from build123d import *

# Parameters (mm, degrees)
EXTRUDE_1_DEPTH = 7.65
SKETCH_2_R      = 6
EXTRUDE_2_DEPTH = 30
FILLET_1_R      = 0.6


with BuildPart() as part:
    # 草图1 → 凸台-拉伸1 (new body)
    with BuildSketch(Plane(origin=(0, 0, 0), x_dir=(1, 0, 0), z_dir=(0, 1, 0))):
        Polygon((6.921438907, -7.752011575), (10.174158408, 2.118136136), (3.252719501, 9.870147711), (-6.921438907, 7.752011575), (-10.174158408, -2.118136136), (-3.252719501, -9.870147711), align=None)
    extrude(amount=EXTRUDE_1_DEPTH)

    # 草图2 → 凸台-拉伸2 (add)
    with BuildSketch(Plane.XZ):
        Circle(SKETCH_2_R)
    extrude(amount=EXTRUDE_2_DEPTH)

    # 圆角1
    fillet_1_edges = [part.edges().sort_by_distance(p)[0] for p in [
        (6.713438955, 7.65, -5.994141924),
        (-1.834359703, 7.65, -8.811079643),
        (-8.547798657, 7.65, -2.81693772),
        (-6.713438955, 7.65, 5.994141924),
        (1.834359703, 7.65, 8.811079643),
        (8.547798657, 7.65, 2.81693772),
    ]]
    fillet(fillet_1_edges, radius=FILLET_1_R)


solid = part.part
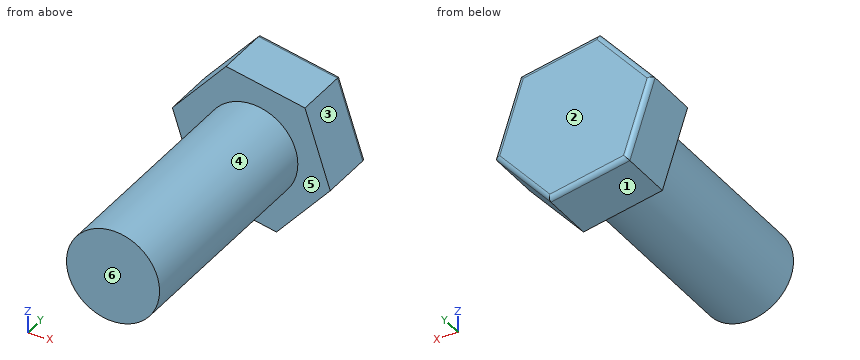
Can you work these out from the model? Positions are in its coordinate system, mm. Face numbers are marked on the shaded views. A direction names the side the tool comes from. Round coordinates to 2 decimals unless told otherwise and drop trailing zeros. Order: outer loops, then holes, each group sorted by start corner. A loop starts at its lowest first (then second) coordinate and runs counter-clockwise, first axis right, second up. Notation, with made-up numbers: (72.5, 40.5) -> (124.5, 40.5) arc R20 ccw to (124.5, 47.5) -> close; hole circle Ø10 at (16, 37.5). An arc over 180 degrees is marked (long way). Write each question's results on one line, items separated by ' | '. Start each with the question number.
Item 1: Will these pins go through, and if not, where does the flat tip stop? pin 1 (1 mm diameter, centred on y = -24, z = 2, fed in from +X); pin 2 (8 mm diameter, centred on y = -17, z = -5, fed in from +X); pin 3 (2 mm diameter, centred on x = -5, y = -4, fed in from -Z).
Item 2: Thinking about a two-plate mould opening in Z: for the marked faces 1, 2, 3 and 4, which applies, +Z half, -Z half, draft (parallel to the pull), parting line (faces both ways), or undercut?
Item 3: Which directions (+Z, -Z, +X, -X, +Y, -Y) give clear straight access to the entire face, cutting with the end or side of a thin tool? Please do the marked faces 5 and 6.
Item 4: If we section it at A-A, the plane y = 2: Write out the boundary of the cut face in (x, z), then the cut area to 3 significant figures.
Item 5: Please list where these lines run through material, in increasing order: L1, parallel to Y at x = 8, z = 2.75; L2, parallel to X at y = -26, z = 1.25; L3, parallel to Z at x = 6, y = 5.
Item 6: If we section it at B-B, the plane y = -24.5: Write out the boundary of the cut face in (x, z), then the cut area to 3 significant figures.
Results:
1) pin 1: stops at x = 5.81 | pin 2: stops at x = 5.92 | pin 3: stops at z = -4.47
2) face 1: -Z half | face 2: draft | face 3: +Z half | face 4: parting line
3) face 5: -Y | face 6: +Z, -Z, +X, -X, -Y
4) outline: (-10.17, 2.12) -> (-6.92, -7.75) -> (3.25, -9.87) -> (10.17, -2.12) -> (6.92, 7.75) -> (-3.25, 9.87) -> close | area: 281 mm2
5) L1: y = 0 to 7.65 | L2: x = -5.87 to 5.87 | L3: z = -6.79 to 7.94
6) outline: circle Ø12 at (0, 0) | area: 113 mm2
